Geometry: final body of the model. Coordinates: model frame, mm. Face numbers are marked on the shaded views. A direction names the side the tool comes from. Give positions to 0.01 mm unless a question says otherwise; leave off trailing zeros. Write each loop counter-clockwise with the first axis right and the second up, starting at its lowest first coordinate (ties: lowest second). Pieces come first, ordered by that corner, then holes.
Q1. Draft query along X for the marked faces 1, 2 and 3. Return one class per face: pulls with the +X half, pulls with the -X half, needs draft (parallel to the pull), parting line crosses it, or undercut.
Q2. Cut plane C-C on x = 35. Return the cut outline in (y, z).
Q3. Cut plane B-B on z = -11.5. Return the cut outline in (x, y).
Q4. Reachability of the marked faces 4 and 5 from +Z, -Z, +X, -X, +Y, -Y: full face, straight path, thin tool, end or side. Return the list, or none.
Q5. Pin query (flat end, axial travel): pin 1 (0.5 mm diameter, centred on x = 126, y = 26, fed in from -Z); pin 2 (10 mm diameter, centred on x = 45, z = -56.5, fed in from +Y); pin 3 (0.8 mm diameter, centred on x = 126, y = 26.5, fed in from +Z). Return the tip coordinate at first contact, or that it passes through.
Q6. Cut plane A-A on y = 19. Return the cut outline in (x, z).
Q7. Line query: L1, parallel to X at y = 24.5, z = -20.5; L2, parallel to Z at x = 105.5, y = 11; L3, parallel to Y at x = 7, z = -15. Output: solid intervals per line, ascending.
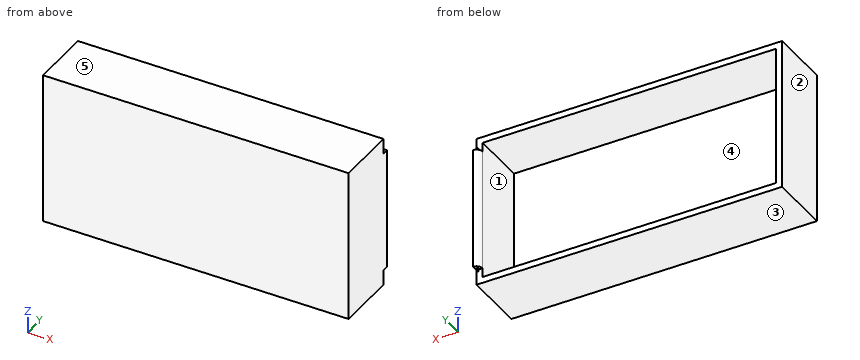
```python
from build123d import *

# Parameters (mm, degrees)
SKETCH1_W                = 127
SKETCH1_H                = 63.5
BOSS_EXTRUDE1_DEPTH      = 25.4
SHELL1_T                 = -2.54
BOSS_EXTRUDE2_DEPTH      = 25.4
BOSS_EXTRUDE2_DEPTH_BACK = 25.4
BOSS_EXTRUDE3_DEPTH      = 1.27
BOSS_EXTRUDE3_DEPTH_BACK = 52.07
SKETCH3_R                = 0.3175


with BuildPart() as part:
    # Sketch1 → Boss-Extrude1 (new body)
    with BuildSketch(Plane(origin=(0, 0, 0), x_dir=(1, 0, 0), z_dir=(0, 1, 0))):
        with Locations((63.5, 31.75)):
            Rectangle(SKETCH1_W, SKETCH1_H)
    extrude(amount=BOSS_EXTRUDE1_DEPTH)

    # Shell1
    shell1_openings = [part.faces().sort_by_distance(p)[0] for p in [
        (63.5, 25.4, -31.75),
    ]]
    offset(amount=SHELL1_T, openings=shell1_openings, kind=Kind.INTERSECTION)

    # Sketch2 → Boss-Extrude2 (add, two sides: drawn at the far end of the back side and taken through both)
    with BuildSketch(Plane.XY.offset(-31.75).offset(-BOSS_EXTRUDE2_DEPTH_BACK)):
        with BuildLine():
            Line((124.46, 25.4), (127, 25.4))
            Line((127, 25.4), (127, 27.94))
            ThreePointArc((127, 27.94), (125.203948776, 27.196051224), (124.46, 25.4))
        make_face()
    extrude(amount=BOSS_EXTRUDE2_DEPTH + BOSS_EXTRUDE2_DEPTH_BACK)

    # Sketch3 → Boss-Extrude3 (add, two sides: drawn at the far end of the back side and taken through both)
    with BuildSketch(Plane.XY.offset(-6.35).offset(-BOSS_EXTRUDE3_DEPTH_BACK)):
        with Locations((126.0475, 26.3525)):
            Circle(SKETCH3_R)
    extrude(amount=BOSS_EXTRUDE3_DEPTH + BOSS_EXTRUDE3_DEPTH_BACK)


solid = part.part
```
Data:
1. face 1: undercut
1. face 2: pulls with the -X half
1. face 3: needs draft
2. outline: (0, -63.5) - (25.4, -63.5) - (25.4, -60.96) - (2.54, -60.96) - (2.54, -2.54) - (25.4, -2.54) - (25.4, 0) - (0, 0) - close
3. outline: (0, 0) - (127, 0) - (127, 27.94) arc R2.54 ccw to (124.46, 25.4) - (124.46, 2.54) - (2.54, 2.54) - (2.54, 25.4) - (0, 25.4) - close
4. face 4: +Y
4. face 5: +Z, +X, -X, +Y, -Y
5. pin 1: stops at z = -58.42
5. pin 2: stops at y = 25.4
5. pin 3: stops at z = -5.08
6. outline: (0, -63.5) - (127, -63.5) - (127, 0) - (0, 0) - close; hole (2.54, -60.96) - (124.46, -60.96) - (124.46, -2.54) - (2.54, -2.54) - close
7. L1: x = 0 to 2.54, 124.46 to 127
7. L2: z = -63.5 to -60.96, -2.54 to 0
7. L3: y = 0 to 2.54
